Can you work these out from the drawing? Everything is in mm from the part's minimum corner. A direction names the side the tool comes from. Give positions to 0.01 mm unless a question says otherwise; leave off trailing zeros. Order: outer loops, then holes, each group sorted by start corner. A loop starts at its lowest first (then second) coordinate and runs counter-clockwise, first axis right, second up. Notation, with made-up numbers: M 12,22.25 L 25,22.25 A9 cw 25,27.25 Z; hole C -13.75,61.25 d1. An arc over 180 degrees is marked long. Use a Markdown table: item, result. Add a question column.
Item 1: Suppose I cut it at C-C on z = 2.5. Write out the boundary of the cut face in (x, y).
Item 2: Suppose I cut it at D-D on y = 9. Write out the boundary of the cut face in (x, z), plus the area to 3 significant figures.
Item 3: If I drill on L1, parallel to X at y = 6, z = 3.5; L2, parallel to Z at x = 6, y = 5; L3, parallel to Y at x = 68, z = 3.5, over which ranges is the centre line in solid material (lowest first)? Write a range as from..to.
Item 4: For the marked faces 5, 6, 7 and 8, which set-ups out of +Z, -Z, +X, -X, +Y, -Y let a thin tool reach every point of the face, with its end or its side?
Item 5: Suppose I cut it at B-B on x = 41. Write out the boundary of the cut face in (y, z).
Item 6: I'm going to push flat-ended pins straight in: pin 1 Ø3 at (x, y) = (40, 33.5) entering from -Z; pin 2 Ø6.5 at (x, z) = (6, 7.5) entering from -Y. Where does each tip first touch, or does it pass through?
Item 7: Suppose I cut it at A-A on z = 7.5. Write out the boundary of the cut face in (x, y), plus the area to 3 significant figures.
Item 8: If we mould it in two halves opening along X, with no side actions, what happens to the marked faces 1, 2, 3 and 4? For each: released by +X, released by -X, zero draft, split by the parting line, or undercut.
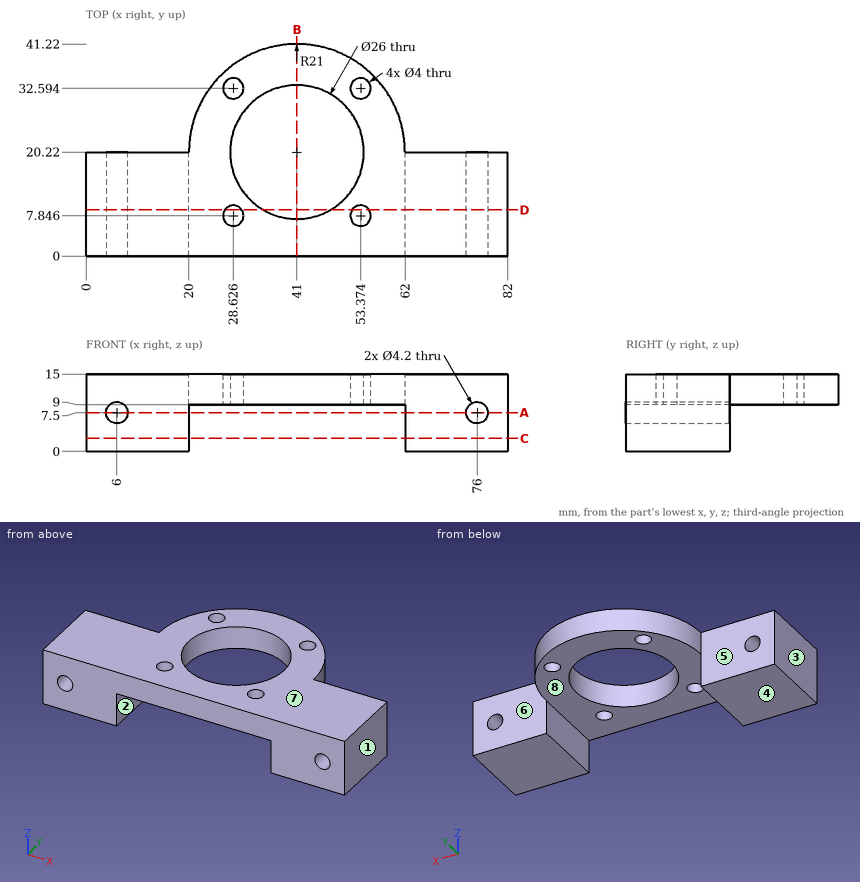
Findings below:
| question | item | result |
|---|---|---|
| 1 | outline | M 0,0 L 20,0 L 20,20.22 L 0,20.22 Z; M 62,0 L 82,0 L 82,20.22 L 62,20.22 Z |
| 2 | outline | M 0,0 L 20,0 L 20,9 L 26.99,9 L 26.99,15 L 0,15 Z; M 30.26,9 L 34.43,9 L 34.43,15 L 30.26,15 Z; M 47.57,9 L 51.74,9 L 51.74,15 L 47.57,15 Z; M 55.01,9 L 62,9 L 62,0 L 82,0 L 82,15 L 55.01,15 Z; hole C 6,7.5 d4.2; hole C 76,7.5 d4.2 |
| 2 | area | 706 mm^2 |
| 3 | L1 | x = 0..20, 62..82 |
| 3 | L2 | z = 0..5.4, 9.6..15 |
| 3 | L3 | y = 0..20.22 |
| 4 | face 5 | +Z, -Z, -X, +Y |
| 4 | face 6 | +Z, -Z, +X, +Y |
| 4 | face 7 | +Z, +X, -X, +Y, -Y |
| 4 | face 8 | -Z, +Y, -Y |
| 5 | outline | M 0,9 L 7.22,9 L 7.22,15 L 0,15 Z; M 33.22,9 L 41.22,9 L 41.22,15 L 33.22,15 Z |
| 6 | pin 1 | stops at z = 9 |
| 6 | pin 2 | stops at y = 0 |
| 7 | outline | M 0,0 L 3.9,0 L 3.9,20.22 L 0,20.22 Z; M 8.1,0 L 20,0 L 20,20.22 L 8.1,20.22 Z; M 62,0 L 73.9,0 L 73.9,20.22 L 62,20.22 Z; M 78.1,0 L 82,0 L 82,20.22 L 78.1,20.22 Z |
| 7 | area | 639 mm^2 |
| 8 | face 1 | released by +X |
| 8 | face 2 | undercut |
| 8 | face 3 | released by -X |
| 8 | face 4 | zero draft |
